The listing builds one solid part. Answer for the finished solid, in the listing's coordinates (mm). Round coordinates to 2 decimals unless told otherwise and drop trailing zeros. Loops run counter-clockwise (first coordinate to the right, second up) from the corner with the lowest first, then second, coordinate; pieces in that order, holes last. Notation, with made-up numbers: (25.5, -37.75) -> (67.5, -37.75) arc R13 cw to (67.5, -31.75) -> close; hole circle Ø2 at (-11, -39.75). An arc over 180 degrees is marked (long way). Write each question's results on one line, items separated by ' | '. Start each with the question number.
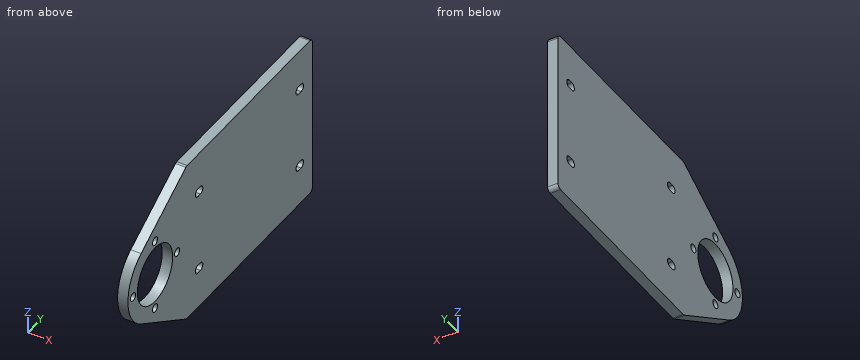
from build123d import *

# Parameters (mm, degrees)
SKETCH1_W           = 80
SKETCH1_H           = 100
SKETCH1_R           = 21.5
SKETCH1_R_2         = 14
SKETCH1_R_3         = 2
BOSS_EXTRUDE1_DEPTH = 5
FILLET1_R           = 2


with BuildPart() as part:
    # Sketch1 → Boss-Extrude1 (new body)
    with BuildSketch(Plane(origin=(0, 0, 0), x_dir=(0, 0, -1), z_dir=(1, 0, 0))):
        Rectangle(SKETCH1_W, SKETCH1_H)
        with BuildLine():
            ThreePointArc((22, -39), (20, -37), (18, -39))
            Line((18, -39), (18, -41))
            ThreePointArc((18, -41), (20, -43), (22, -41))
            Line((22, -41), (22, -39))
        make_face(mode=Mode.SUBTRACT)
        with BuildLine():
            ThreePointArc((-22, 39), (-20, 37), (-18, 39))
            Line((-18, 39), (-18, 41))
            ThreePointArc((-18, 41), (-20, 43), (-22, 41))
            Line((-22, 41), (-22, 39))
        make_face(mode=Mode.SUBTRACT)
        with BuildLine():
            Line((22, 41), (22, 39))
            ThreePointArc((22, 39), (20, 37), (18, 39))
            Line((18, 39), (18, 41))
            ThreePointArc((18, 41), (20, 43), (22, 41))
        make_face(mode=Mode.SUBTRACT)
        with BuildLine():
            Line((-22, -41), (-22, -39))
            ThreePointArc((-22, -39), (-20, -37), (-18, -39))
            Line((-18, -39), (-18, -41))
            ThreePointArc((-18, -41), (-20, -43), (-22, -41))
        make_face(mode=Mode.SUBTRACT)
        with BuildLine():
            Line((40, -50), (-40, -50))
            Line((-40, -50), (-18.452584301, -86.034134882))
            ThreePointArc((-18.452584301, -86.034134882), (-5.72361064, -54.275852702), (21.5, -75))
            ThreePointArc((21.5, -75), (20.724147298, -80.72361064), (18.452584301, -86.034134882))
            Line((18.452584301, -86.034134882), (40, -50))
        make_face()
        with Locations((0, -75)):
            Circle(SKETCH1_R)
        with Locations((0, -75)):
            Circle(SKETCH1_R_2, mode=Mode.SUBTRACT)
        with Locations((17.5, -75)):
            Circle(SKETCH1_R_3, mode=Mode.SUBTRACT)
        with Locations((0, -92.5)):
            Circle(SKETCH1_R_3, mode=Mode.SUBTRACT)
        with Locations((-17.5, -75)):
            Circle(SKETCH1_R_3, mode=Mode.SUBTRACT)
        with Locations((0, -57.5)):
            Circle(SKETCH1_R_3, mode=Mode.SUBTRACT)
    extrude(amount=BOSS_EXTRUDE1_DEPTH)

    # Fillet1
    fillet1_edges = [part.edges().sort_by_distance(p)[0] for p in [
        (2.5, -50, -40),
        (2.5, -50, 40),
        (2.5, 50, 40),
        (2.5, 50, -40),
    ]]
    fillet(fillet1_edges, radius=FILLET1_R)


solid = part.part
Item 1: The part is cut by section C-C, the plane z = 8.5. Give the vertices of the cut face in (x, y), plus the area to 4 significant figures.
Item 2: The part is cut by section D-D, the plane y = -75. Give the vertices of the cut face in (x, z).
Item 3: The part is cut by section B-B, the plane x = 2.55. Give the number of separate pieces and of enclosed holes in the cut face, plus the area to 3 significant figures.
Item 4: Straight lines are drawn through the part: L1, parallel to Y at x = 1.55, z = 0; L2, parallel to Z at x = 2.3, y = -39.5; L3, parallel to Y at x = 1.95, z = -1.5. For each, find the intervals that lie inside material, in ascending order. Write a range as [from, to].
Item 5: Each of these flat-tipped pins is pushed along its axis until it touches: pin 1 Ø3.5 at (y, z) = (-57.5, 0) entering from +X; pin 2 Ø1.5 at (x, z) = (3.5, 24.5) entering from -Y; pin 3 Ø1.5 at (x, z) = (3.5, 17) entering from -Y. Where does it stop, or does it pass through?
Item 6: The part is cut by section A-A, the plane y = -92.5. Give the vertices of the cut face in (x, z).
Report:
1) outline: (0, -94.75) -> (5, -94.75) -> (5, -86.12) -> (0, -86.12) -> close; (0, -63.88) -> (5, -63.88) -> (5, 50) -> (0, 50) -> close | area: 612.5 mm2
2) outline: (0, -25.05) -> (5, -25.05) -> (5, -19.5) -> (0, -19.5) -> close; (0, -15.5) -> (5, -15.5) -> (5, -14) -> (0, -14) -> close; (0, 14) -> (5, 14) -> (5, 15.5) -> (0, 15.5) -> close; (0, 19.5) -> (5, 19.5) -> (5, 25.05) -> (0, 25.05) -> close
3) separate pieces: 1 | enclosed holes: 9 | area: 9,630 mm2
4) L1: y = [-96.5, -94.5], [-90.5, -89], [-61, -59.5], [-55.5, 50] | L2: z = [-40, -22], [-18, 18], [22, 40] | L3: y = [-96.45, -93.82], [-91.18, -88.92], [-61.08, -58.82], [-56.18, 50]
5) pin 1: passes through | pin 2: stops at y = -77.18 | pin 3: stops at y = -89.08
6) outline: (0, -12.49) -> (5, -12.49) -> (5, -2) -> (0, -2) -> close; (0, 2) -> (5, 2) -> (5, 12.49) -> (0, 12.49) -> close
